from build123d import *

# Parameters (mm, degrees)
ESBO_O2_R         = 3
EXTRUS_O1_DEPTH   = 10
EXTRUS_O1_TAPER   = 3
CIRPATTERN1_COUNT = 8


with BuildPart() as part:
    # Esbo_o1 → Revolu_o1 (revolve)
    with BuildSketch(Plane.XY, mode=Mode.PRIVATE) as revolu_o1_sk:
        Polygon((0, 10.5), (82, 10.5), (82, 29.5), (92, 29.5), (92, 42.5), (82, 43.5), (82, 44.5), (0, 44.5), (0, 43.5), (-12, 42.5), (-12, 35.5), (-3.89618766, 35.5), (-3.89618766, 29.5), (0, 29.5), align=None)
    revolve(revolu_o1_sk.sketch.rotate(Axis((0, 0, 0), (1, 0, 0)), 90), axis=Axis((0, 0, 0), (1, 0, 0)))

    # Esbo_o2 → Extrus_o1 (add)
    with BuildSketch(Plane(origin=(92, 0, 0), x_dir=(0, 0, -1), z_dir=(1, 0, 0))):
        with Locations((0, 36)):
            Circle(ESBO_O2_R)
    extrus_o1 = extrude(amount=EXTRUS_O1_DEPTH, taper=EXTRUS_O1_TAPER)

    # CirPattern1: Extrus_o1 ×8 about axis
    cirpattern1_axis = Axis((0, 0, 0), (1, 0, 0))
    for i in range(1, CIRPATTERN1_COUNT):
        add(extrus_o1.rotate(cirpattern1_axis, i * 360 / CIRPATTERN1_COUNT))


solid = part.part
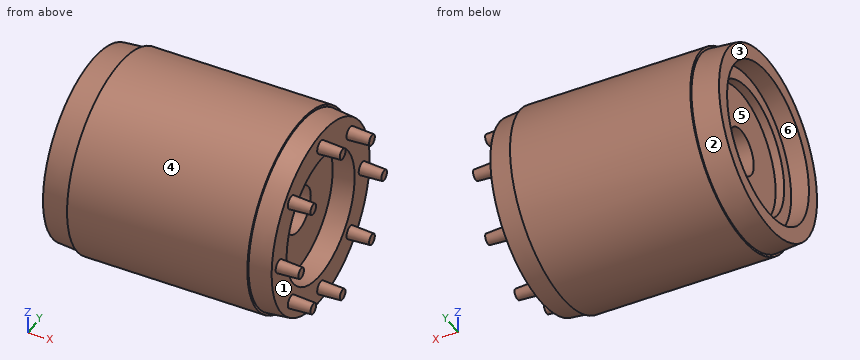
Can you work these out from the model? Positions are in its coordinate system, mm. Face numbers are marked on the shaded views. A direction names the side the tool comes from. Round coordinates to 2 decimals unless told otherwise and drop trailing zeros. Order: outer loops, then holes, each group sorted by start corner. A loop starts at its lowest first (then second) coordinate and runs counter-clockwise, first axis right, second up. Notation, with made-up numbers: (-21, 71) - (-15, 71) arc R25 cw to (-15, 103) - close; hole circle Ø3 at (67, 5.25). An arc over 180 degrees is marked (long way). Answer in a Markdown table with one row per item.
(1) Please list where these lines run through material, in increasing order: L1, parallel to Y at x = 30, z = 9; L2, parallel to X at y = 17, z = -27; L3, parallel to Z at x = 49.5, y = 3. Write a range as from..to.
From the geometry:
| item | result |
|---|---|
| L1 | y = -43.58..-5.41, 5.41..43.58 |
| L2 | x = -3.9..92 |
| L3 | z = -44.4..-10.06, 10.06..44.4 |
(2) Suppose I cut it at B-B, the plane x = 90.5. Please give me the cut outline in (y, z), plus the area to 3 significant figures.
From the geometry:
| item | result |
|---|---|
| outline | circle Ø85.3 at (0, 0); hole circle Ø59 at (0, 0) |
| area | 2,980 mm2 |
(3) Which directions (+Z, -Z, +X, -X, +Y, -Y) give clear straight access to the entire face, cutting with the end or side of a thin tool? Please do the marked faces 1 and 2.
From the geometry:
| item | result |
|---|---|
| face 1 | +X |
| face 2 | -X |
(4) If we mould it in two halves opening along Y, with no side actions, what happens to the marked faces 3, 4, 5 and 6? For each: released by +Y, released by -Y, zero draft, split by the parting line, or undercut.
From the geometry:
| item | result |
|---|---|
| face 3 | zero draft |
| face 4 | split by the parting line |
| face 5 | undercut |
| face 6 | undercut |
(5) Suppose I cut it at A-A, the plane x = 23.5. Please give me the cut outline in (y, z).
From the geometry:
| item | result |
|---|---|
| outline | circle Ø89 at (0, 0); hole circle Ø21 at (0, 0) |
(6) For P1, Ø4, axis at x = 60, z = 6.5, coming from the -Y side; P2, Ø6, axis at y = 8, z = 2, coming from the +X side; P3, Ø8, axis at x = 87, y = 18, coming from the +Z side, each with a flat end and sliding along its axis, tell me the tip position at first contact or that it passes through.
From the geometry:
| item | result |
|---|---|
| P1 | stops at y = -44.27 |
| P2 | stops at x = 82 |
| P3 | stops at z = 40.72 |
